```python
from build123d import *

# Parameters (mm, degrees)
SKETCH2_R               = 26.5303
SKETCH2_R_2             = 21.3868
BOSS_EXTRUDE1_DEPTH     = 27.0002
CUT_EXTRUDE1_DEPTH      = 47.224716724
CUT_EXTRUDE1_DEPTH_BACK = 47.224716724
SKETCH3_W               = 3.048
SKETCH3_H               = 4.572


with BuildPart() as part:
    # Sketch2 → Boss-Extrude1 (new body)
    with BuildSketch(Plane(origin=(0, 0, 0), x_dir=(0, 0, -1), z_dir=(1, 0, 0))):
        Circle(SKETCH2_R)
        Circle(SKETCH2_R_2, mode=Mode.SUBTRACT)
    extrude(amount=BOSS_EXTRUDE1_DEPTH)

    # Sketch3 → Cut-Extrude1 (cut, two sides: drawn at the far end of the back side and taken through both)
    with BuildSketch(Plane.XY.offset(-CUT_EXTRUDE1_DEPTH_BACK)):
        with Locations((25.4762, 0)):
            Rectangle(SKETCH3_W, SKETCH3_H)
    extrude(amount=CUT_EXTRUDE1_DEPTH + CUT_EXTRUDE1_DEPTH_BACK, mode=Mode.SUBTRACT)


solid = part.part
```
Source: CAD feature listing. Evaluate the final solid. Frame: model axes, mm. A direction names the side the tool comes from. Give positions to 0.01 mm unless a question says otherwise; leave off trailing zeros. Order: outer loops, then holes, each group sorted by start corner. A loop starts at its lowest first (then second) coordinate and runs counter-clockwise, first axis right, second up.
(1) Pull-direction query (Y, two-part tool) for faces 3 (the face through (13.311, 7.969, -25.305)), 4 (the face through (27, -22, -2)), 5 (the face through (25, 2.286, -24)), 6 (the face through (25, -2.286, 24)); classes: +Y half, -Y half, draft (parallel to the pull), parting line (faces both ways), or undercut.
(2) Section query D-D (y = 23.5). Return the cut outline in (x, z).
(3) Section query C-C (x = 10.25). Return the cut outline in (y, z).
(4) Section query A-A (y = 0). Return the cut outline in (x, z).
(5) Contact query for flat-ended pins moving along their axis: P1, Ø2, axis at x = 21, y = 9.5, coming from the -Z side; P2, Ø2.5, axis at y = 0.5, z = -23.5, coming from the +X side; P3, Ø4, axis at x = 22, y = -2.5, coming from the +Z side; P4, Ø1.5, axis at y = -14, z = 19, coming from the -X side. Output: stop coordinate, or through.
(6) Section query B-B (z = 0). Return the cut outline in (x, y), plus the area to 3 significant figures.
(7) Material intervals for line 1 along Y through (x, z) = (13, 0); line 2 along Y through (x, z) = (13.5, 16); line 3 along Z through (x, y) = (15, 10.5), sorted ascending.
(8) Access query for faces 1 (the face through (27, 22, -2)), 2 (the face through (25, 2.286, 24)). Directions: +Z, -Z, +X, -X, +Y, -Y. A direction counts if a zero-diameter tool reaches every point of the face in a straight line with its end or side. Return the directions, or none.
Outcome:
1. face 3: parting line
1. face 4: draft
1. face 5: undercut
1. face 6: undercut
2. outline: (0, -12.31) - (27, -12.31) - (27, 12.31) - (0, 12.31) - close
3. outline: circle Ø53.06 at (0, 0); hole circle Ø42.77 at (0, 0)
4. outline: (0, -26.53) - (23.95, -26.53) - (23.95, -21.39) - (0, -21.39) - close; (0, 21.39) - (23.95, 21.39) - (23.95, 26.53) - (0, 26.53) - close
5. P1: stops at z = -25.13
5. P2: stops at x = 23.95
5. P3: stops at z = 26.53
5. P4: stops at x = 0
6. outline: (0, -26.53) - (27, -26.53) - (27, -21.39) - (0, -21.39) - close; (0, 21.39) - (27, 21.39) - (27, 26.53) - (0, 26.53) - close
6. area: 278 mm2
7. line 1: y = -26.53 to -21.39, 21.39 to 26.53
7. line 2: y = -21.16 to -14.19, 14.19 to 21.16
7. line 3: z = -24.36 to -18.63, 18.63 to 24.36
8. face 1: +Z, -Z, +X, +Y, -Y
8. face 2: +Z, -Z, +X
